CAD build for the part. Positions are in the model's coordinates, mm. Face numbers are marked on the shaded views. Coordinates: 2 decimals unless noted, no trailing zeros. Order: outer loops, then holes, each group sorted by start corner. A loop starts at its lowest first (then second) coordinate and runs counter-clockwise, first axis right, second up. Notation, with made-up numbers: (-5.75, 35.25) - (6.25, 35.25) arc R27 cw to (6.25, 71.25) - close; hole circle Ø7 at (15, 81.25). An arc over 180 degrees is marked (long way). Write each question's results on one line, items separated by ' | '. Start each with the question number.
Q1. Band-saw the part on B-B, the plane z = 2.5. Write the cut outline in (x, y).
Q2. Band-saw the part on A-A, the plane y = -2.5. Write the cut outline in (x, z), then the cut area to 3 significant figures.
Q3. Wall check: probe 1 along X at (y, z) = (-1.4, 4.6); probe 2 along X at (y, z) = (-4.3, 4.75); probe 3 along Y at (x, z) = (8, 0.5). Give the ranges that are in metal, low to high.
Q4. Pull direction X, two halves, no side cores. Call the marked faces 1, 2 and 3: released by +X, released by -X, zero draft, split by the parting line, or undercut.
Q5. Pin check, flat tip, straight feed: P1, Ø1.5, axis at x = -47.5, y = -2.5, coming from the -Z side. Stop position of the tip, or through.
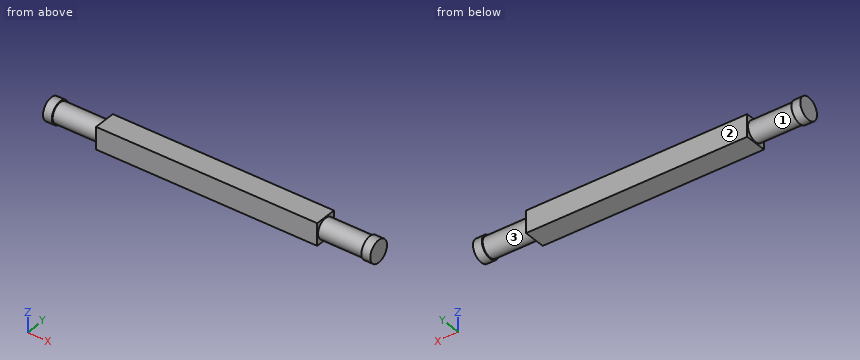
```python
from build123d import *

# Parameters (mm, degrees)
ESBO_O1_W                = 50
ESBO_O1_H                = 5
RESSALTO_EXTRUS_O1_DEPTH = 5
ESBO_O2_R                = 2.25
RESSALTO_EXTRUS_O2_DEPTH = 10
ESBO_O3_R                = 2.5
RESSALTO_EXTRUS_O3_DEPTH = 2


with BuildPart() as part:
    # Esboço1 → Ressalto-extrusão1 (new body)
    with BuildSketch(Plane.XY):
        with Locations((-25, -2.5)):
            Rectangle(ESBO_O1_W, ESBO_O1_H)
    extrude(amount=RESSALTO_EXTRUS_O1_DEPTH)

    # Esboço2 → Ressalto-extrusão2 (add)
    with BuildSketch(Plane.ZY.offset(50)):
        with Locations(Location((2.5, -2.5, 0), (0, 0, 180))):
            Circle(ESBO_O2_R)
    ressalto_extrus_o2 = extrude(amount=RESSALTO_EXTRUS_O2_DEPTH)

    # Esboço3 → Ressalto-extrusão3 (add)
    with BuildSketch(Plane.ZY.offset(60)):
        with Locations((2.5, -2.5)):
            Circle(ESBO_O3_R)
    ressalto_extrus_o3 = extrude(amount=RESSALTO_EXTRUS_O3_DEPTH)

    # Espelhar1: Ressalto-extrusão2, Ressalto-extrusão3 across plane
    add(ressalto_extrus_o2.mirror(Plane.ZY.offset(25)))
    add(ressalto_extrus_o3.mirror(Plane.ZY.offset(25)))


solid = part.part
```
Results below:
1) outline: (-62, -5) - (-60, -5) - (-60, -4.75) - (-50, -4.75) - (-50, -5) - (0, -5) - (0, -4.75) - (10, -4.75) - (10, -5) - (12, -5) - (12, 0) - (10, 0) - (10, -0.25) - (0, -0.25) - (0, 0) - (-50, 0) - (-50, -0.25) - (-60, -0.25) - (-60, 0) - (-62, 0) - close
2) outline: (-62, 0) - (-60, 0) - (-60, 0.25) - (-50, 0.25) - (-50, 0) - (0, 0) - (0, 0.25) - (10, 0.25) - (10, 0) - (12, 0) - (12, 5) - (10, 5) - (10, 4.75) - (0, 4.75) - (0, 5) - (-50, 5) - (-50, 4.75) - (-60, 4.75) - (-60, 5) - (-62, 5) - close | area: 360 mm²
3) probe 1: x = -62 to -60, -50 to 0, 10 to 12 | probe 2: x = -50 to 0 | probe 3: y = -3.53 to -1.47
4) face 1: undercut | face 2: zero draft | face 3: undercut
5) P1: stops at z = 0
